Print and shaded views of the part. All mm, measured from the part's lowest x, y and z. A direction names the side the tool comes from. Coordinates: 2 decimals unless noted, no trailing zeros. Loops run counter-clockwise (first coordinate to the right, second up) from the corner with the lowest first, then second, coordinate; pieces in that order, holes last. Notation, with made-up numbers: M 68.5,0.5 L 110.5,0.5 A5 ccw 110.5,5.5 Z; hole C -28,-10.5 d4. An arc over 180 degrees is marked long. Use a Markdown table: item, result. Add a question column.
1) Tool access for the marked faces 4, 5 and 6: list every direction of +Z, -Z, +X, -X, +Y, -Y with a clear straight run to the whole face (end or side of a thin tool).
2) Pull direction X, two halves, no side cores. Call the marked faces 1, 2 and 3: released by +X, released by -X, zero draft, split by the parting line, or undercut.
3) Band-saw the part on A-A (y = 41). List the corners of the cut face in (x, z).
4) Band-saw the part on C-C (x = 11.5). List the corners of the cut face in (y, z) (1 decimal).
5) Band-saw the part on B-B (y = 20). List the corners of the cut face in (x, z).
6) Band-saw the part on D-D (y = 33). List the corners of the cut face in (x, z).
7) Pin check, flat tips, straight feed: pin 1 Ø1 at (x, z) = (9, 4) entering from -Y; pin 2 Ø12 at (x, y) = (22.5, 29.5) entering from +Z; pin 3 Ø4 at (x, y) = (16.5, 25) entering from +Z. Stop position of each tip, or through.
8) Wall check: probe 1 along Z at (x, y) = (22.75, 41); probe 2 along Y at (x, z) = (23.25, 4); probe 3 along X at (y, z) = (3.5, 6.75). Give the ranges that are in metal, low to high. Write a range as from..to.
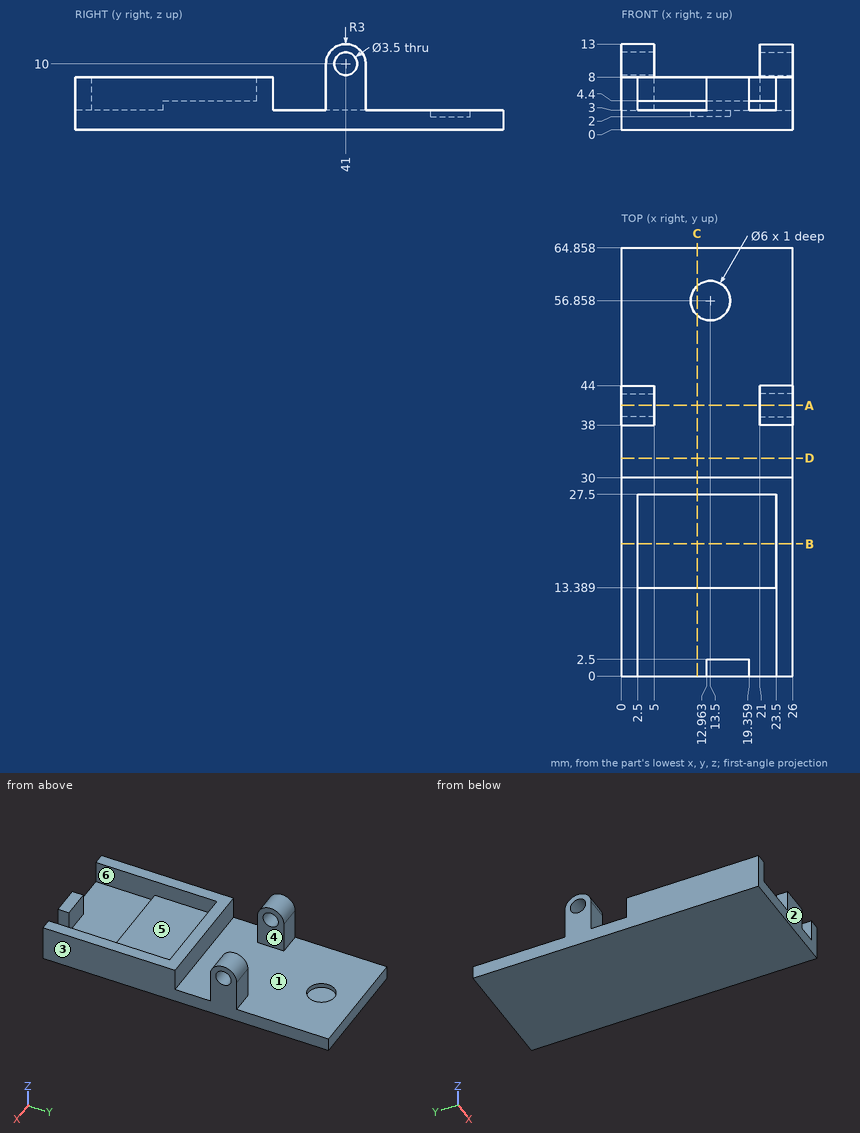
Entries:
| question | item | result |
|---|---|---|
| 1 | face 4 | +Z, +Y |
| 1 | face 5 | +Z |
| 1 | face 6 | +Z, -Y |
| 2 | face 1 | undercut |
| 2 | face 2 | zero draft |
| 2 | face 3 | released by +X |
| 3 | outline | M 0,0 L 26,0 L 26,8.25 L 21,8.25 L 21,3 L 5,3 L 5,8.25 L 0,8.25 Z; M 0,11.75 L 5,11.75 L 5,13 L 0,13 Z; M 21,11.75 L 26,11.75 L 26,13 L 21,13 Z |
| 4 | outline | M 0,0 L 64.9,0 L 64.9,3 L 59.1,3 L 59.1,2 L 54.6,2 L 54.6,3 L 30,3 L 30,8 L 27.5,8 L 27.5,4.4 L 13.4,4.4 L 13.4,3 L 0,3 Z |
| 5 | outline | M 0,0 L 26,0 L 26,8 L 23.5,8 L 23.5,4.4 L 2.5,4.4 L 2.5,8 L 0,8 Z |
| 6 | outline | M 0,0 L 26,0 L 26,3 L 0,3 Z |
| 7 | pin 1 | y = 13.39 |
| 7 | pin 2 | z = 8 |
| 7 | pin 3 | z = 4.4 |
| 8 | probe 1 | 0..8.25, 11.75..13 |
| 8 | probe 2 | 13.39..30, 38..44 |
| 8 | probe 3 | 0..2.5, 23.5..26 |
